```python
from build123d import *

# Parameters (mm, degrees)
PAD_DEPTH    = 55
SKETCH001_R  = 1.6
POCKET_DEPTH = 3.001
FILLET_R     = 3
FILLET001_R  = 5


with BuildPart() as part:
    # Sketch → Pad (new body, symmetric)
    with BuildSketch(Plane.XZ):
        Polygon((-41, -3), (-41, 37), (-38, 37), (-38, 0), (38, 0), (38, 37), (41, 37), (41, -3), align=None)
    extrude(amount=PAD_DEPTH, both=True)

    # Sketch001 (on Face4 of Pad) → Pocket (cut, through all)
    with BuildSketch(Plane(origin=(0, 0, 0), x_dir=(-1, 0, 0), z_dir=(0, 0, 1))):
        with Locations((-30, 50)):
            Circle(SKETCH001_R)
        with Locations((30, 50)):
            Circle(SKETCH001_R)
        with Locations((-30, -50)):
            Circle(SKETCH001_R)
        with Locations((30, -50)):
            Circle(SKETCH001_R)
        with Locations((-14, 22.5)):
            Circle(SKETCH001_R)
        with Locations((14, 22.5)):
            Circle(SKETCH001_R)
    extrude(amount=-POCKET_DEPTH, mode=Mode.SUBTRACT)

    # Fillet
    fillet_edges = [part.edges().sort_by_distance(p)[0] for p in [
        (-41, 0, -3),
        (41, 0, -3),
    ]]
    fillet(fillet_edges, radius=FILLET_R)

    # Fillet001
    fillet001_edges = [part.edges().sort_by_distance(p)[0] for p in [
        (39.5, -55, 37),
        (-39.5, -55, 37),
        (-39.5, 55, 37),
        (39.5, 55, 37),
    ]]
    fillet(fillet001_edges, radius=FILLET001_R)


solid = part.part
```
CAD build for the part. Positions are in the model's coordinates, mm. A direction names the side the tool comes from. Coordinates: 2 decimals unless noted, no trailing zeros. Order: outer loops, then holes, each group sorted by start corner. A loop starts at its lowest first (then second) coordinate and runs counter-clockwise, first axis right, second up. Notation, with made-up numbers: (49.25, 80.25) - (77.25, 80.25) arc R15 ccw to (77.25, 87.25) - close; hole circle Ø5 at (56.25, 89.5). An arc over 180 degrees is marked (long way). Answer in a Markdown table with one row per item.
1. Slice it at C-C, the plane z = 6. List the corners of the cut face in (x, y), then the cut area to 3 significant figures.
Answer:
| item | result |
|---|---|
| outline | (-41, -55) - (-38, -55) - (-38, 55) - (-41, 55) - close; (38, -55) - (41, -55) - (41, 55) - (38, 55) - close |
| area | 660 mm² |
2. Slice it at A-A, the plane x = -30. List the corners of the cut face in (y, z).
Answer:
| item | result |
|---|---|
| outline | (-55, -3) - (-51.6, -3) - (-51.6, 0) - (-55, 0) - close; (-48.4, -3) - (48.4, -3) - (48.4, 0) - (-48.4, 0) - close; (51.6, -3) - (55, -3) - (55, 0) - (51.6, 0) - close |
3. Slice it at B-B, the plane y = -22.5. List the corners of the cut face in (x, z).
Answer:
| item | result |
|---|---|
| outline | (-41, 0) arc R3 ccw to (-38, -3) - (-15.6, -3) - (-15.6, 0) - (-38, 0) - (-38, 37) - (-41, 37) - close; (-12.4, -3) - (12.4, -3) - (12.4, 0) - (-12.4, 0) - close; (15.6, -3) - (38, -3) arc R3 ccw to (41, 0) - (41, 37) - (38, 37) - (38, 0) - (15.6, 0) - close |
4. Drill centre lines: L1, parallel to Y at x = -30, z = -1; L2, parallel to Y at x = -14, z = -1.8; L3, parallel to X at y = -19, z = 3.5. Where is each one in solid material? Low to high. Write a range as from..to.
Answer:
| item | result |
|---|---|
| L1 | -55..-51.6, -48.4..48.4, 51.6..55 |
| L2 | -55..-24.1, -20.9..55 |
| L3 | -41..-38, 38..41 |
5. Pull direction Y, two halves, no side cores. Call faces 3 (the face through (-28.4, -50.07, -1.48)), 4 (the face through (39, -1, 37)), 5 (the face through (40, -54, 35)): +Y half, -Y half, draft (parallel to the pull), parting line (faces both ways), or undercut.
Answer:
| item | result |
|---|---|
| face 3 | undercut |
| face 4 | draft |
| face 5 | -Y half |
6. Flat gauge pin, fed straight in: P1, Ø5, axis at x = -30, y = -50, coming from the +Z side. Where does the tip first touch, or does it go through?
Answer:
| item | result |
|---|---|
| P1 | z = 0 |
7. 3-axis set-ups, long thin cutter, end or side, ignore diameter. For faces 1 (the face through (-28.4, 49.93, -1.48)), 2 (the face through (-38, -1, 19)): which of +Z, -Z, +X, -X, +Y, -Y reach the whole face in a straight line?
Answer:
| item | result |
|---|---|
| face 1 | +Z, -Z |
| face 2 | +Z, +Y, -Y |
8. Slice it at D-D, the plane x = 14. List the corners of the cut face in (y, z), then the cut area to 3 significant figures.
Answer:
| item | result |
|---|---|
| outline | (-55, -3) - (-24.1, -3) - (-24.1, 0) - (-55, 0) - close; (-20.9, -3) - (55, -3) - (55, 0) - (-20.9, 0) - close |
| area | 320 mm² |
